Read the model definition and answer for the solid it produces. Units are mm, in the model's axes. A direction names the side the tool comes from. Give positions to 0.01 mm unless a question says otherwise; leave off trailing zeros. Loops run counter-clockwise (first coordinate to the right, second up) from the corner with the lowest first, then second, coordinate; pieces in that order, holes last.
(1) Find section A-A, the plane y = 0. Write down the section's boundary in (x, z).
(2) Which of the six approach directions +Z, -Z, +X, -X, +Y, -Y give full straight-line access (tool end or side, diameter ignored) to faces 1 (the face through (5.5, -3.1, 0.2)), 2 (the face through (2, -2, 1)), 3 (the face through (2.712, 9.423, 9.489)), 4 (the face through (2.712, 5.803, -10.072))?
(3) Find section D-D, the plane z = -9. Write down the section's boundary in (x, y).
(4) Determine the mould class of faces 5 (the face through (2.712, 7.75, 10.957)), 6 (the face through (2.712, 8.911, 7.464)), 7 (the face through (0, 3, 0)), 8 (the face through (2.71, 5.61, 12.14)) for opening direction Z: pulls with the +Z half, pulls with the -Z half, needs draft (parallel to the pull), parting line crosses it, or undercut.
(5) Straight lines are drawn through the part: probe 1 along Y at (x, z) = (3.2, 0); probe 2 along Y at (x, z) = (0.65, 0); probe 3 along Z at (x, y) = (1.45, -10.75). For each, find the intervals that lie inside material, in ascending order.
(6) Find section C-C, the plane y = -9. Write down the section's boundary in (x, z), then the cut area to 3 significant figures.
(7) Find section B-B, the plane z = 0. Write down the section's boundary in (x, y).
(8) Each of these flat-tipped pins is pushed along its axis until it touches: P1, Ø1.5, axis at x = 4.5, z = -9.5, coming from the -Y side; P2, Ø2, axis at x = 4.5, y = -7.5, coming from the -Z side; P3, Ø3, axis at x = 1.5, y = -5.5, coming from the -Z side. Where does it stop, or does it pass through?
```python
from build123d import *

# Parameters (mm, degrees)
BASPROSKE_W             = 7
BASPROSKE_H             = 15
TOOTHCUT_DEPTH          = 23.338307904
TEETHCUTS_COUNT         = 18
TEETHCUTS_ANGLE         = 340
BORSKE_R                = 2.5
BORE_DEPTH              = 50.0000508
CROQUIS1_R              = 2.9
CORTAR_EXTRUIR1_DEPTH   = 10
CROQUIS4_R              = 3.489132724
SALIENTE_EXTRUIR1_DEPTH = 2
CROQUIS5_R              = 1.9
CORTAR_EXTRUIR3_DEPTH   = 5
CROQUIS6_R              = 21.972687295
CORTAR_EXTRUIR4_DEPTH   = 1.5


with BuildPart() as part:
    # BasProSke → Base-Revolve (revolve)
    with BuildSketch(Plane(origin=(0, 0, 0), x_dir=(1, 0, 0), z_dir=(0, 1, 0)), mode=Mode.PRIVATE) as base_revolve_sk:
        with Locations((3.5, 7.5)):
            Rectangle(BASPROSKE_W, BASPROSKE_H)
    revolve(base_revolve_sk.sketch.rotate(Axis((-10, 0, 0), (1, 0, 0)), 180), axis=Axis((-10, 0, 0), (1, 0, 0)))

    # TooCutSke → ToothCut (cut, through all)
    with BuildSketch(Plane(origin=(0, 0, 0), x_dir=(0, 0, -1), z_dir=(1, 0, 0))):
        with BuildLine():
            ThreePointArc((0.759974923, 11.599129886), (0, 11.624), (-0.759974923, 11.599129886))
            ThreePointArc((-0.759974923, 11.599129886), (-1.229186471, 13.354767823), (-2.254227748, 14.855339189))
            ThreePointArc((-2.254227748, 14.855339189), (0, 15.0254), (2.254227748, 14.855339189))
            ThreePointArc((2.254227748, 14.855339189), (1.229186471, 13.354767823), (0.759974923, 11.599129886))
        make_face()
    toothcut = extrude(amount=TOOTHCUT_DEPTH, mode=Mode.SUBTRACT)

    # TeethCuts: ToothCut ×18 about axis
    teethcuts_axis = Axis((-10, 0, 0), (1, 0, 0))
    for i in range(1, TEETHCUTS_COUNT):
        add(toothcut.rotate(teethcuts_axis, i * TEETHCUTS_ANGLE / (TEETHCUTS_COUNT - 1)), mode=Mode.SUBTRACT)

    # BorSke → Bore (cut, symmetric)
    with BuildSketch(Plane(origin=(0, 0, 0), x_dir=(0, 0, -1), z_dir=(1, 0, 0))):
        with Locations(Location((0, 0, 0), (0, 0, 180))):
            Circle(BORSKE_R)
    extrude(amount=BORE_DEPTH, both=True, mode=Mode.SUBTRACT)

    # Croquis1 → Cortar-Extruir1 (cut)
    with BuildSketch(Plane(origin=(7, 0, 0), x_dir=(0, 0, -1), z_dir=(1, 0, 0))):
        Circle(CROQUIS1_R)
    extrude(amount=-CORTAR_EXTRUIR1_DEPTH, mode=Mode.SUBTRACT)

    # Croquis4 → Saliente-Extruir1 (add, through all)
    with BuildSketch(Plane.ZY.offset(-2)):
        Circle(CROQUIS4_R)
    extrude(amount=SALIENTE_EXTRUIR1_DEPTH)

    # Croquis5 → Cortar-Extruir3 (cut)
    with BuildSketch(Plane(origin=(2, 0, 0), x_dir=(0, 0, -1), z_dir=(1, 0, 0))):
        Circle(CROQUIS5_R)
    extrude(amount=-CORTAR_EXTRUIR3_DEPTH, mode=Mode.SUBTRACT)

    # Croquis6 → Cortar-Extruir4 (cut)
    with BuildSketch(Plane(origin=(7, 0, 0), x_dir=(0, 0, -1), z_dir=(1, 0, 0))):
        Circle(CROQUIS6_R)
    extrude(amount=-CORTAR_EXTRUIR4_DEPTH, mode=Mode.SUBTRACT)


solid = part.part
```
Entries:
1. outline: (0, -15) - (5.5, -15) - (5.5, -2.9) - (2, -2.9) - (2, -1.9) - (0, -1.9) - close; (0, 1.9) - (2, 1.9) - (2, 2.9) - (5.5, 2.9) - (5.5, 15) - (0, 15) - close
2. face 1: +Z, -Z, +X, +Y, -Y
2. face 2: +X
2. face 3: +X, -X, +Y
2. face 4: +X, -X
3. outline: (0, -9.15) - (5.5, -9.15) - (5.5, 9.15) - (0, 9.15) - close
4. face 5: pulls with the +Z half
4. face 6: undercut
4. face 7: needs draft
4. face 8: undercut
5. probe 1: y = -11.62 to -2.9, 2.9 to 11.62
5. probe 2: y = -11.62 to -1.9, 1.9 to 11.62
5. probe 3: z = -7.56 to -4.73, -4.42 to 4.42, 4.73 to 7.56
6. outline: (0, -11.61) - (5.5, -11.61) - (5.5, -8.76) - (0, -8.76) - close; (0, -7.36) - (5.5, -7.36) - (5.5, 7.36) - (0, 7.36) - close; (0, 8.76) - (5.5, 8.76) - (5.5, 11.61) - (0, 11.61) - close
6. area: 112 mm2
7. outline: (0, -11.62) - (5.5, -11.62) - (5.5, -2.9) - (2, -2.9) - (2, -1.9) - (0, -1.9) - close; (0, 1.9) - (2, 1.9) - (2, 2.9) - (5.5, 2.9) - (5.5, 11.62) - (0, 11.62) - close
8. P1: stops at y = -9.72
8. P2: stops at z = -11.4
8. P3: stops at z = -14.22
